```python
from build123d import *

# Parameters (mm, degrees)
BOSS_EXTRUDE1_DEPTH = 2.9972
SKETCH9_R           = 1.397
CUT_EXTRUDE3_DEPTH  = 3.9972
SKETCH10_R          = 1.80975
CUT_EXTRUDE4_DEPTH  = 3.9972
SKETCH11_R          = 1.6
CUT_EXTRUDE5_DEPTH  = 3.9972
SKETCH12_R          = 1.016
CUT_EXTRUDE6_DEPTH  = 3.9972


with BuildPart() as part:
    # Sketch3 → Boss-Extrude1 (new body)
    with BuildSketch(Plane.XY):
        Polygon((38.1, 0), (38.1, -2.9972), (101.6, -2.9972), (101.6, 0), (139.7, 0), (139.7, 5.08), (142.6972, 5.08), (142.6972, 0), (147.7772, 0), (147.7772, 69.85), (142.6972, 69.85), (142.6972, 64.77), (139.7, 64.77), (139.7, 69.85), (101.6, 69.85), (101.6, 72.8472), (38.1, 72.8472), (38.1, 69.85), (0, 69.85), (0, 64.77), (-2.9972, 64.77), (-2.9972, 69.85), (-8.0772, 69.85), (-8.0772, 0), (-2.9972, 0), (-2.9972, 5.08), (0, 5.08), (0, 0), align=None)
    extrude(amount=BOSS_EXTRUDE1_DEPTH)

    # Sketch9 → Cut-Extrude3 (cut, through all)
    with BuildSketch(Plane(origin=(0, 0, 0), x_dir=(-1, 0, 0), z_dir=(0, 0, -1))):
        with Locations((-31.6484, 4.445)):
            Circle(SKETCH9_R)
        with Locations((-108.0516, 65.405)):
            Circle(SKETCH9_R)
        with Locations((-108.0516, 4.445)):
            Circle(SKETCH9_R)
        with Locations((-31.6484, 65.405)):
            Circle(SKETCH9_R)
    extrude(amount=-CUT_EXTRUDE3_DEPTH, mode=Mode.SUBTRACT)

    # Sketch10 → Cut-Extrude4 (cut, through all)
    with BuildSketch(Plane(origin=(0, 0, 0), x_dir=(-1, 0, 0), z_dir=(0, 0, -1))):
        with Locations((-53.1368, 44.48175)):
            Circle(SKETCH10_R)
        with Locations((-34.967367815, 59.34075)):
            Circle(SKETCH10_R)
        with Locations((-87.189767815, 53.40985)):
            Circle(SKETCH10_R)
        with Locations((-103.85425, 59.63285)):
            Circle(SKETCH10_R)
        with Locations((-87.335817815, 25.36825)):
            Circle(SKETCH10_R)
        with Locations((-105.50525, 10.50925)):
            Circle(SKETCH10_R)
        with Locations((-53.28285, 16.44015)):
            Circle(SKETCH10_R)
        with Locations((-36.618367815, 10.21715)):
            Circle(SKETCH10_R)
    extrude(amount=-CUT_EXTRUDE4_DEPTH, mode=Mode.SUBTRACT)

    # Sketch11 → Cut-Extrude5 (cut, through all)
    with BuildSketch(Plane(origin=(0, 0, 0), x_dir=(-1, 0, 0), z_dir=(0, 0, -1))):
        with Locations((-119.38, 58.864027758)):
            Circle(SKETCH11_R)
        with Locations((-120.98, 10.985972242)):
            Circle(SKETCH11_R)
        with Locations((-68.629534614, 15.487902261)):
            Circle(SKETCH11_R)
        with Locations((-68.390649314, 43.386879551)):
            Circle(SKETCH11_R)
        with Locations((-21.50999995, 11.950503851)):
            Circle(SKETCH11_R)
        with Locations((-20.32, 59.840503852)):
            Circle(SKETCH11_R)
        with Locations((-72.629999995, 54.890503798)):
            Circle(SKETCH11_R)
        with Locations((-72.629999966, 26.990503798)):
            Circle(SKETCH11_R)
    extrude(amount=-CUT_EXTRUDE5_DEPTH, mode=Mode.SUBTRACT)

    # Sketch12 → Cut-Extrude6 (cut, through all)
    with BuildSketch(Plane.XY.offset(2.9972)):
        with Locations((10.414, 21.1074)):
            Circle(SKETCH12_R)
        with Locations((10.414, 48.7426)):
            Circle(SKETCH12_R)
        with Locations((41.9862, 21.1074)):
            Circle(SKETCH12_R)
        with Locations((41.9862, 48.7426)):
            Circle(SKETCH12_R)
        with Locations((129.286, 21.1074)):
            Circle(SKETCH12_R)
        with Locations((129.286, 48.7426)):
            Circle(SKETCH12_R)
        with Locations((97.7138, 21.1074)):
            Circle(SKETCH12_R)
        with Locations((97.7138, 48.7426)):
            Circle(SKETCH12_R)
    extrude(amount=-CUT_EXTRUDE6_DEPTH, mode=Mode.SUBTRACT)


solid = part.part
```
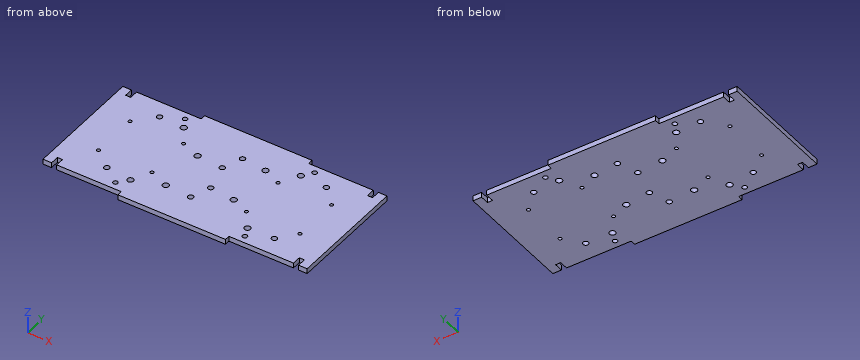
Can you work these out from the model? Positions are in its coordinate system, mm. Give positions to 0.01 mm unless a question says otherwise; leave off trailing zeros. Write each loop counter-clockwise with the first axis right and the second up, starting at its lowest first coordinate (ties: lowest second). Pieces come first, ordered by that corner, then holes. Notation, with made-up numbers: (-21, 3.25) -> (7, 3.25) arc R20 ccw to (7, 14.25) -> close; hole circle Ø11 at (-12, -35.75). An arc over 180 degrees is marked (long way). One line per item, written item: value.
Q1. Imagine slicing it at C-C on z = 1.95. Give the number of separate pieces and of enclosed holes in the cut face, and give its area (3 significant figures).
Results found:
separate pieces: 1
enclosed holes: 28
area: 11,000 mm^2
Q2. Imagine slicing it at A-A on x = 87. Please give me the cut outline in (y, z), and give its area (3 significant figures).
Results found:
outline: (-3, 0) -> (23.59, 0) -> (23.59, 3) -> (-3, 3) -> close; (27.15, 0) -> (51.61, 0) -> (51.61, 3) -> (27.15, 3) -> close; (55.21, 0) -> (72.85, 0) -> (72.85, 3) -> (55.21, 3) -> close
area: 206 mm^2
Q3. Please list where these lines run through material, in increasing order: line 1 (X direction, y = 1, z = 1.2); line 2 (X direction, y = 21, z = 2.5); line 3 (Y direction, x = 42, z = 2.45). Write a range as [from, to].
Results found:
line 1: x = [-8.08, -3], [0, 139.7], [142.7, 147.78]
line 2: x = [-8.08, 9.4], [11.42, 40.98], [43, 96.7], [98.72, 128.28], [130.3, 147.78]
line 3: y = [-3, 20.09], [22.12, 47.73], [49.76, 72.85]
Q4. Imagine slicing it at B-B on x = 14. Please give me the cut outline in (y, z).
Results found:
outline: (0, 0) -> (69.85, 0) -> (69.85, 3) -> (0, 3) -> close
Q5. For P1, Ø3, axis at x = 53.14, y = 44.48, coming from the -Z side; P2, Ø4.5, axis at x = 108.05, y = 4.44, coming from the -Z side; P3, Ø0.9, axis at x = -1.5, z = 2, coming from the -Y side, each with a flat end and sliding along its axis, tell me the tip position at first contact or that it passes through.
Results found:
P1: passes through
P2: stops at z = 0
P3: stops at y = 5.08
